Source: CAD feature listing. Evaluate the final solid. Frame: model axes, mm. Face numbers are marked on the shaded views. A direction names the side the tool comes from. Coordinates: 2 decimals unless noted, no trailing zeros. Loops run counter-clockwise (first coordinate to the right, second up) from the corner with the lowest first, then second, coordinate; pieces in that order, holes last. Notation, with made-up numbers: (61.5, 63.5) -> (104.5, 63.5) arc R14 cw to (104.5, 74.5) -> close; hole circle Ø5 at (80.25, 78.25). An arc over 180 degrees is marked (long way). Answer as CSV lines item,"result".
from build123d import *

# Parameters (mm, degrees)
BOSS_EXTRUDE1_DEPTH     = 20.5
SKETCH2_W               = 88
SKETCH2_H               = 51
SKETCH2_R               = 7.75
CUT_EXTRUDE1_DEPTH      = 66.463730416
CUT_EXTRUDE1_DEPTH_BACK = 66.463730416
SKETCH4_W               = 10.25
SKETCH4_H               = 15.6
BOSS_EXTRUDE2_DEPTH     = 25
CUT_EXTRUDE2_REACH      = 69.756
SKETCH5_R               = 1.25
SKETCH6_R               = 2.25
CUT_EXTRUDE3_DEPTH      = 29.3
CUT_EXTRUDE4_REACH      = 88.338
CUT_EXTRUDE5_DEPTH      = 3.5


with BuildPart() as part:
    # Sketch1 → Boss-Extrude1 (new, symmetric)
    with BuildSketch(Plane.YZ):
        with BuildLine():
            Line((-53, -32.5), (-17, -32.5))
            Line((-17, -32.5), (-17, -25.5))
            Line((-17, -25.5), (0, -25.5))
            ThreePointArc((0, -25.5), (25.5, 0), (0, 25.5))
            Line((0, 25.5), (-17, 25.5))
            Line((-17, 25.5), (-17, 32.5))
            Line((-17, 32.5), (-53, 32.5))
            Line((-53, 32.5), (-53, 29))
            Line((-53, 29), (-24, 29))
            Line((-24, 29), (-24, -29))
            Line((-24, -29), (-53, -29))
            Line((-53, -29), (-53, -32.5))
        make_face()
        with BuildLine():
            Line((-3.644391878, -9.312271895), (-6.200961894, -13.740381057))
            Line((-6.200961894, -13.740381057), (-8.799038106, -12.240381057))
            Line((-8.799038106, -12.240381057), (-6.242468089, -7.812271895))
            ThreePointArc((-6.242468089, -7.812271895), (-8.660254038, -5), (-9.886859967, -1.5))
            Line((-9.886859967, -1.5), (-15, -1.5))
            Line((-15, -1.5), (-15, 1.5))
            Line((-15, 1.5), (-9.886859967, 1.5))
            ThreePointArc((-9.886859967, 1.5), (-8.660254038, 5), (-6.242468089, 7.812271895))
            Line((-6.242468089, 7.812271895), (-8.799038106, 12.240381057))
            Line((-8.799038106, 12.240381057), (-6.200961894, 13.740381057))
            Line((-6.200961894, 13.740381057), (-3.644391878, 9.312271895))
            ThreePointArc((-3.644391878, 9.312271895), (0, 10), (3.644391878, 9.312271895))
            Line((3.644391878, 9.312271895), (6.200961894, 13.740381057))
            Line((6.200961894, 13.740381057), (8.799038106, 12.240381057))
            Line((8.799038106, 12.240381057), (6.242468089, 7.812271895))
            ThreePointArc((6.242468089, 7.812271895), (10, 0), (6.242468089, -7.812271895))
            Line((6.242468089, -7.812271895), (8.799038106, -12.240381057))
            Line((8.799038106, -12.240381057), (6.200961894, -13.740381057))
            Line((6.200961894, -13.740381057), (3.644391878, -9.312271895))
            ThreePointArc((3.644391878, -9.312271895), (0, -10), (-3.644391878, -9.312271895))
        make_face(mode=Mode.SUBTRACT)
    extrude(amount=BOSS_EXTRUDE1_DEPTH, both=True)

    # Sketch2 → Cut-Extrude1 (cut, two sides)
    with BuildSketch(Plane(origin=(0, 0, 0), x_dir=(0, 1, 0), z_dir=(0, 0, 1))) as cut_extrude1_sk:
        with Locations((-14, 0)):
            Rectangle(SKETCH2_W, SKETCH2_H)
        with BuildLine():
            Line((-10, 15.5), (25, 15.5))
            Line((25, 15.5), (25, 20.5))
            Line((25, 20.5), (-32.5, 20.5))
            ThreePointArc((-32.5, 20.5), (-53, 0), (-32.5, -20.5))
            Line((-32.5, -20.5), (25, -20.5))
            Line((25, -20.5), (25, -15.5))
            Line((25, -15.5), (-10, -15.5))
            Line((-10, -15.5), (-10, 15.5))
        make_face(mode=Mode.SUBTRACT)
        with Locations(Location((-41, 0, 0), (0, 0, 270))):
            Circle(SKETCH2_R)
    extrude(amount=CUT_EXTRUDE1_DEPTH, mode=Mode.SUBTRACT)
    extrude(cut_extrude1_sk.sketch, amount=-CUT_EXTRUDE1_DEPTH_BACK, mode=Mode.SUBTRACT)

    # Sketch4 → Boss-Extrude2 (add)
    with BuildSketch(Plane.XZ.offset(24)):
        with Locations((15.375, 3.4)):
            Rectangle(SKETCH4_W, SKETCH4_H)
    extrude(amount=BOSS_EXTRUDE2_DEPTH)

    # Sketch5 → Cut-Extrude2 (cut, up to next)
    with BuildSketch(Plane(origin=(0, 0, -4.4), x_dir=(1, 0, 0), z_dir=(0, 0, -1)), mode=Mode.PRIVATE) as cut_extrude2_sk1:
        with Locations(Location((14, 46, 0), (0, 0, 270))):
            Circle(SKETCH5_R)
    cut_extrude2_tool1 = extrude(cut_extrude2_sk1.sketch, amount=-CUT_EXTRUDE2_REACH, mode=Mode.PRIVATE) & part.part
    # Sketch5 → Cut-Extrude2 (cut, up to next)
    with BuildSketch(Plane(origin=(0, 0, -4.4), x_dir=(1, 0, 0), z_dir=(0, 0, -1)), mode=Mode.PRIVATE) as cut_extrude2_sk2:
        with Locations(Location((14, 36, 0), (0, 0, 180))):
            Circle(SKETCH5_R)
    cut_extrude2_tool2 = extrude(cut_extrude2_sk2.sketch, amount=-CUT_EXTRUDE2_REACH, mode=Mode.PRIVATE) & part.part
    add(cut_extrude2_tool1.solids().sort_by_distance((14, -46, -4.4))[0], mode=Mode.SUBTRACT)
    add(cut_extrude2_tool2.solids().sort_by_distance((14, -36, -4.4))[0], mode=Mode.SUBTRACT)

    # Sketch6 → Cut-Extrude3 (cut)
    with BuildSketch(Plane(origin=(0, 0, -32.5), x_dir=(1, 0, 0), z_dir=(0, 0, -1))):
        with Locations(Location((14, 46, 0), (0, 0, 270))):
            Circle(SKETCH6_R)
        with Locations(Location((14, 36, 0), (0, 0, 90))):
            Circle(SKETCH6_R)
    extrude(amount=-CUT_EXTRUDE3_DEPTH, mode=Mode.SUBTRACT)

    # Sketch7 → Cut-Extrude4 (cut, up to next)
    with BuildSketch(Plane.XY.offset(32.5), mode=Mode.PRIVATE) as cut_extrude4_sk1:
        with BuildLine():
            Line((-12.304878049, -39.397222885), (-12.304878049, -48.89634033))
            Line((-12.304878049, -48.89634033), (-20.5, -48.89634033))
            Line((-20.5, -48.89634033), (-20.5, -41.884242803))
            Line((-20.5, -41.884242803), (-20.5, -29.602755078))
            ThreePointArc((-20.5, -29.602755078), (-19.791785251, -31.497638771), (-18.041662968, -32.512145713))
            ThreePointArc((-18.041662968, -32.512145713), (-13.927029708, -34.916291372), (-12.304878049, -39.397222885))
        make_face()
    cut_extrude4_tool1 = extrude(cut_extrude4_sk1.sketch, amount=-CUT_EXTRUDE4_REACH, mode=Mode.PRIVATE) & part.part
    add(cut_extrude4_tool1.solids().sort_by_distance((-16.657353, -41.093277, 32.5))[0], mode=Mode.SUBTRACT)

    # Sketch9 → Cut-Extrude5 (cut)
    with BuildSketch(Plane(origin=(0, 0, -32.5), x_dir=(1, 0, 0), z_dir=(0, 0, -1))):
        with BuildLine():
            Line((20.5, 49.298437427), (20.5, 24))
            ThreePointArc((20.5, 24), (19.540037651, 26.945860787), (17.028761689, 28.760555398))
            ThreePointArc((17.028761689, 28.760555398), (13.209828458, 31.520187417), (11.75, 36))
            Line((11.75, 36), (11.75, 49.298437427))
            Line((11.75, 49.298437427), (20.5, 49.298437427))
        make_face()
    extrude(amount=-CUT_EXTRUDE5_DEPTH, mode=Mode.SUBTRACT)


solid = part.part
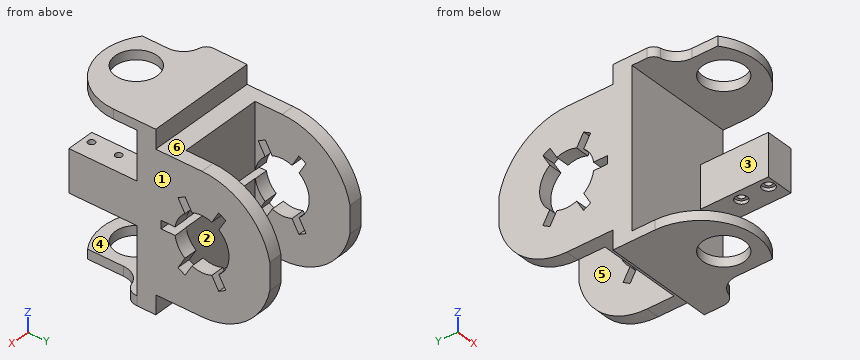
(1) Pin query (flat end, axial travel): pin 1 Ø5.5 at (x, y) = (-6.5, -12.5) entering from +Z; pin 2 Ø2 at (x, z) = (-3, 28) entering from +Y; pin 3 Ø0.9 at (x, z) = (6.5, 0.5) entering from +Y; pin 4 Ø5 at (x, y) = (-4.5, -6.5) entering from +Z. Return the tip coordinate at first contact, or that it passes through.
Computed values:
pin 1,"z = 25.5"
pin 2,"y = -17"
pin 3,"y = -15"
pin 4,"through"
(2) Draft query along X for the marked faces 1, 2 and 3. Return one class per face: released by +X, released by -X, zero draft, split by the parting line, or undercut.
Computed values:
face 1,"released by +X"
face 2,"undercut"
face 3,"released by -X"
(3) Cut plane D-D (y = 14). Return the cut outline in (x, z), then the cut area to 3 significant figures.
Computed values:
outline,"(-20.5, -21.31) -> (-15.5, -21.31) -> (-15.5, 21.31) -> (-20.5, 21.31) -> close; (15.5, -21.31) -> (20.5, -21.31) -> (20.5, 21.31) -> (15.5, 21.31) -> close"
area,"426 mm^2"
(4) Cut plane A-A (x = 0). Return the cut outline in (y, z).
Computed values:
outline,"(-53, -32.5) -> (-48.75, -32.5) -> (-48.75, -29) -> (-53, -29) -> close; (-53, 29) -> (-48.75, 29) -> (-48.75, 32.5) -> (-53, 32.5) -> close; (-33.25, -32.5) -> (-17, -32.5) -> (-17, -25.5) -> (-10, -25.5) -> (-10, -1.5) -> (-15, -1.5) -> (-15, 1.5) -> (-10, 1.5) -> (-10, 25.5) -> (-17, 25.5) -> (-17, 32.5) -> (-33.25, 32.5) -> (-33.25, 29) -> (-24, 29) -> (-24, -29) -> (-33.25, -29) -> close"
(5) Cut plane B-B (y = -46). Return the cut outline in (x, z), then the cut area to 3 significant figures.
Computed values:
outline,"(-15.43, -32.5) -> (-5.92, -32.5) -> (-5.92, -29) -> (-15.43, -29) -> close; (-12.3, 29) -> (-5.92, 29) -> (-5.92, 32.5) -> (-12.3, 32.5) -> close; (5.92, -32.5) -> (11.75, -32.5) -> (11.75, -29) -> (5.92, -29) -> close; (5.92, 29) -> (15.43, 29) -> (15.43, 32.5) -> (5.92, 32.5) -> close; (10.25, -4.4) -> (11.75, -4.4) -> (11.75, -3.2) -> (12.75, -3.2) -> (12.75, 11.2) -> (10.25, 11.2) -> close; (15.25, -3.2) -> (16.25, -3.2) -> (16.25, -4.4) -> (20.5, -4.4) -> (20.5, 11.2) -> (15.25, 11.2) -> close"
area,"228 mm^2"
(6) Access query for the marked faces 4, 5 and 6. Directions: +Z, -Z, +X, -X, +Y, -Y. A direction counts if a zero-diameter tool reaches every point of the face in a straight line with its end or side. Return the directions, or none.
Computed values:
face 4,"+X, -X, -Y"
face 5,"+Z, -Z, +Y"
face 6,"+Z, +X, -X, +Y"
(7) Material intervals for L1, parallel to Z at x = -16, y = -31; L2, parallel to Z at x = 16.5, y = -40.5; L3, parallel to Y at x = 0, z = 30.7, sorted ascending. Write a range as [from, to].
Computed values:
L1,"[-32.5, -29], [29, 32.5]"
L2,"[-4.4, 11.2], [29, 32.5]"
L3,"[-53, -48.75], [-33.25, -17]"
(8) Cut plane C-C (z = 22.5). Return the cut outline in (x, y), then the cut area to 3 significant figures.
Computed values:
outline,"(-20.5, -24) -> (20.5, -24) -> (20.5, 12) -> (15.5, 12) -> (15.5, -10) -> (-15.5, -10) -> (-15.5, 12) -> (-20.5, 12) -> close"
area,"794 mm^2"
